Here's how the part is built. I have some questions about the finished solid (model axes, mm). A direction names the side the tool comes from. Coordinates: 2 decimals unless noted, no trailing zeros. Write each loop counter-clockwise with the first axis right and the second up, starting at its lowest first coordinate (ties: lowest second). Pieces come first, ordered by that corner, then holes. Notation, with made-up numbers: (-40, 86) -> (-28, 86) arc R29 cw to (-28, 118) -> close; hole circle Ø11 at (-19.5, 34.5). An arc over 180 degrees is marked (long way). Use a Markdown table: item, result. Add a question column.
Item 1: On a 3-axis mill with a long thin cutter (end or side, diameter ignored), from which of +Z, -Z, +X, -X, +Y, -Y can I reach the whole of each face in a straight line? I mean faces 1 (the cylindrical face through (-22.106, 22.185, -21.846)), 2 (the flat face through (1, 0, 1)). Say none if no direction works.
Item 2: Imagine slicing it at C-C, the plane x = 0. Write out the boundary of the cut face in (y, z) (3 decimals), and give its area (3 significant figures).
Item 3: Will these pins go through, and if not, where does the flat tip stop? pin 1 Ø3 at (y, z) = (6, -6.5) entering from -X; pin 2 Ø12 at (x, y) = (2, 35.5) entering from +Z.
Item 4: Imagine slicing it at A-A, the plane x = -9. Write out the boundary of the cut face in (y, z), and give its area (3 significant figures).
Item 5: If we mould it in two halves opening along Z, with no side actions, what happens to faces 3 (the flat face through (-17, 45, -26)), 4 (the cylindrical face through (-34.147, 1.479, -20.708)), 5 (the cylindrical face through (-17.1, 24.3, 6.8))? For each: pulls with the +Z half, pulls with the -Z half, needs draft (parallel to the pull), parting line crosses it, or undercut.
Item 6: If I drill on line 1 along Y through (x, z) = (-6, 12.5); line 2 along Z through (x, y) = (0, 0.6) (3 decimals); line 3 along X through (y, z) = (36, -12.5), over which ranges is the centre line in solid material (lowest first)? Write a range as from..to.
Item 7: Imagine slicing it at B-B, the plane z = 0. Write out the boundary of the cut face in (x, y), and give its area (3 significant figures).
Item 8: Imagine slicing it at D-D, the plane y = 28.5. Write out the boundary of the cut face in (x, z).
Autodesk Inventor part; units mm, degrees
ref_plane "YZ Plane" through (0, 0, 0) normal (1, 0, 0) x (0, 1, 0)
ref_plane "XZ Plane" through (0, 0, 0) normal (0, 1, 0) x (-1, 0, 0)
ref_plane "XY Plane" through (0, 0, 0) normal (0, 0, 1) x (1, 0, 0)
sketch "Sketch1" plane through (0, 0, 0) normal (0, 1, 0) x (-1, 0, 0)
  circle A0 centre (0, 0) radius 44.45
  circle A1 centre (0, -41.275) radius 1.6
  circle A2 centre (35.7452, -20.6375) radius 1.6
  circle A3 centre (-35.7452, -20.6375) radius 1.6
  circle A4 centre (0, 41.275) radius 1.6
  circle A5 centre (35.7452, 20.6375) radius 1.6
  circle A6 centre (-35.7452, 20.6375) radius 1.6
  arc A7 (28.0281, -10.5398) -> (10.5398, -28.0281) centre (12.7279, -12.7279) ccw
  arc A8 (10.5398, -28.0281) -> (28.0281, -10.5398) centre (6.4322, -6.4322) ccw
extrude "Extrusion1" add sketch "Sketch1" along normal blind 45
sketch "Sketch2" plane through (0, 45, 0) normal (0, 1, 0) x (1, 0, 0)
  arc A0 (-28.0281, 10.5398) -> (-10.5398, 28.0281) centre (-12.7279, 12.7279) ccw
  circle A1 centre (-12.7279, 12.7279) radius 20.011
  circle A2 centre (0, 0) radius 44.45
extrude "Extrusion2" cut sketch "Sketch2" against normal blind 42
properties part number "Potting_Jig_Internal"
Ans:
| question | item | result |
|---|---|---|
| 1 | face 1 | +Y, -Y |
| 1 | face 2 | +Z, -Z, +X, -X, -Y |
| 2 | outline | (0, -44.45) -> (3, -44.45) -> (3, -42.875) -> (0, -42.875) -> close; (0, -39.675) -> (3, -39.675) -> (3, -28.169) -> (45, -28.169) -> (45, -21.496) -> (0, -21.496) -> close; (0, -3.96) -> (45, -3.96) -> (45, 2.714) -> (3, 2.714) -> (3, 39.675) -> (0, 39.675) -> close; (0, 42.875) -> (3, 42.875) -> (3, 44.45) -> (0, 44.45) -> close |
| 2 | area | 755 mm^2 |
| 3 | pin 1 | stops at x = -32.17 |
| 3 | pin 2 | stops at z = 5.28 |
| 4 | outline | (0, -43.53) -> (3, -43.53) -> (3, -32.39) -> (45, -32.39) -> (45, -27.73) -> (0, -27.73) -> close; (0, 2.27) -> (45, 2.27) -> (45, 6.93) -> (3, 6.93) -> (3, 43.53) -> (0, 43.53) -> close |
| 4 | area | 563 mm^2 |
| 5 | face 3 | needs draft |
| 5 | face 4 | undercut |
| 5 | face 5 | parting line crosses it |
| 6 | line 1 | y = 0..3 |
| 6 | line 2 | z = -44.45..-42.875, -39.675..-21.496, -3.96..39.675, 42.875..44.45 |
| 6 | line 3 | x = -32.74..-27.56, 2.73..7.28 |
| 7 | outline | (-44.45, 0) -> (-21.5, 0) -> (-21.5, 45) -> (-28.17, 45) -> (-28.17, 3) -> (-44.45, 3) -> close; (-3.96, 0) -> (44.45, 0) -> (44.45, 3) -> (2.71, 3) -> (2.71, 45) -> (-3.96, 45) -> close |
| 7 | area | 775 mm^2 |
| 8 | outline | circle Ø40.02 at (-12.73, -12.73); hole (-28.03, -10.54) arc R21.98 ccw to (-10.54, -28.03) arc R15.46 ccw (long way) to start |
